```python
from build123d import *

# Parameters (mm, degrees)
SKETCH_1_W          = 97.1
SKETCH_1_H          = 100
EXTRUDE_1_DEPTH     = 1.25
SKETCH_2_W          = 10
SKETCH_2_H          = 10
EXTRUDE_2_DEPTH     = 2.5
CUT_EXTRUDE_2_DEPTH = 3.5
SKETCH_3_R          = 0.75
CUT_EXTRUDE_1_DEPTH = 3.5
FILLET_1_R          = 0.5
SKETCH_6_W          = 77.1
SKETCH_6_H          = 40
CUT_EXTRUDE_3_DEPTH = 3.5
CHAMFER_1_SIZE      = 5
FILLET_2_R          = 1
CUT_EXTRUDE_4_DEPTH = 3.5


with BuildPart() as part:
    # 草图1 → 凸台-拉伸1 (new body, symmetric)
    with BuildSketch(Plane.XY):
        Rectangle(SKETCH_1_W, SKETCH_1_H)
    extrude(amount=EXTRUDE_1_DEPTH, both=True)

    # 草图2 → 凸台-拉伸2 (add)
    with BuildSketch(Plane.XY.offset(1.25)):
        with Locations((-48.55, -40)):
            Rectangle(SKETCH_2_W, SKETCH_2_H)
        with Locations((-48.55, 40)):
            Rectangle(SKETCH_2_W, SKETCH_2_H)
        with Locations((48.55, -40)):
            Rectangle(SKETCH_2_W, SKETCH_2_H)
        with Locations((48.55, 40)):
            Rectangle(SKETCH_2_W, SKETCH_2_H)
    extrude(amount=-EXTRUDE_2_DEPTH)

    # 草图5 → 切除-拉伸2 (cut, through all)
    with BuildSketch(Plane.XY.offset(1.25)):
        Polygon((-38.5, 50), (-38.5, 45), (-36, 45), (-36, 35), (-38.5, 35), (-38.5, 30), (38.5, 30), (38.5, 35), (36, 35), (36, 45), (38.5, 45), (38.5, 50), align=None)
        Polygon((-38.5, -50), (-38.5, -45), (-36, -45), (-36, -35), (-38.5, -35), (-38.5, -30), (38.5, -30), (38.5, -35), (36, -35), (36, -45), (38.5, -45), (38.5, -50), align=None)
    extrude(amount=-CUT_EXTRUDE_2_DEPTH, mode=Mode.SUBTRACT)

    # 草图3 → 切除-拉伸1 (cut, through all)
    with BuildSketch(Plane.XY.offset(1.25)):
        with Locations((-48.55, 34.25)):
            Circle(SKETCH_3_R)
        with Locations((-48.55, 45.75)):
            Circle(SKETCH_3_R)
        with Locations((-48.55, -34.25)):
            Circle(SKETCH_3_R)
        with Locations((-48.55, -45.75)):
            Circle(SKETCH_3_R)
        with Locations((48.55, -34.25)):
            Circle(SKETCH_3_R)
        with Locations((48.55, -45.75)):
            Circle(SKETCH_3_R)
        with Locations((48.55, 34.25)):
            Circle(SKETCH_3_R)
        with Locations((48.55, 45.75)):
            Circle(SKETCH_3_R)
        with Locations((-38.5, 45.75)):
            Circle(SKETCH_3_R)
        with Locations((-38.5, 34.25)):
            Circle(SKETCH_3_R)
        with Locations((-37.75, 30)):
            Circle(SKETCH_3_R)
        with Locations((-37.75, -30)):
            Circle(SKETCH_3_R)
        with Locations((-38.5, -34.25)):
            Circle(SKETCH_3_R)
        with Locations((-38.5, -45.75)):
            Circle(SKETCH_3_R)
        with Locations((38.5, -45.75)):
            Circle(SKETCH_3_R)
        with Locations((38.5, -34.25)):
            Circle(SKETCH_3_R)
        with Locations((37.75, -30)):
            Circle(SKETCH_3_R)
        with Locations((37.75, 30)):
            Circle(SKETCH_3_R)
        with Locations((38.5, 34.25)):
            Circle(SKETCH_3_R)
        with Locations((38.5, 45.75)):
            Circle(SKETCH_3_R)
    extrude(amount=-CUT_EXTRUDE_1_DEPTH, mode=Mode.SUBTRACT)

    # 圆角1
    fillet_1_edges = [part.edges().sort_by_distance(p)[0] for p in [
        (36, 45, 0),
        (36, 35, 0),
        (-36, 35, 0),
        (-36, 45, 0),
        (-36, -45, 0),
        (-36, -35, 0),
        (36, -35, 0),
        (36, -45, 0),
        (-53.55, -35, 0),
        (-53.55, -45, 0),
        (-53.55, 45, 0),
        (-53.55, 35, 0),
        (53.55, -45, 0),
        (53.55, -35, 0),
        (53.55, 35, 0),
        (53.55, 45, 0),
    ]]
    fillet(fillet_1_edges, radius=FILLET_1_R)

    # 草图6 → 切除-拉伸3 (cut, through all)
    with BuildSketch(Plane.XY.offset(1.25)):
        Rectangle(SKETCH_6_W, SKETCH_6_H)
    extrude(amount=-CUT_EXTRUDE_3_DEPTH, mode=Mode.SUBTRACT)

    # 倒角1
    chamfer_1_edges = [part.edges().sort_by_distance(p)[0] for p in [
        (-38.55, -20, 0),
        (-38.55, 20, 0),
        (38.55, 20, 0),
        (38.55, -20, 0),
    ]]
    chamfer(chamfer_1_edges, length=CHAMFER_1_SIZE)

    # 圆角2
    fillet_2_edges = [part.edges().sort_by_distance(p)[0] for p in [
        (33.55, -20, 0),
        (-33.55, -20, 0),
        (-38.55, 15, 0),
        (-38.55, -15, 0),
        (38.55, 15, 0),
        (38.55, -15, 0),
        (-33.55, 20, 0),
        (33.55, 20, 0),
    ]]
    fillet(fillet_2_edges, radius=FILLET_2_R)

    # 草图7 → 切除-拉伸4 (cut, through all)
    with BuildSketch(Plane.XY.offset(1.25)):
        with BuildLine():
            Line((-44.525, -42), (-44.525, 42))
            ThreePointArc((-44.525, 42), (-43.525, 43), (-42.525, 42))
            Line((-42.525, 42), (-42.525, -42))
            ThreePointArc((-42.525, -42), (-43.525, -43), (-44.525, -42))
        make_face()
        with BuildLine():
            Line((44.525, -42), (44.525, 42))
            ThreePointArc((44.525, 42), (43.525, 43), (42.525, 42))
            Line((42.525, 42), (42.525, -42))
            ThreePointArc((42.525, -42), (43.525, -43), (44.525, -42))
        make_face()
    extrude(amount=-CUT_EXTRUDE_4_DEPTH, mode=Mode.SUBTRACT)


solid = part.part
```
Design review of the part built by this model. Coordinates are the model's own, in mm. A direction names the side the tool comes from. Round coordinates to 2 decimals unless told otherwise and drop trailing zeros. Order: outer loops, then holes, each group sorted by start corner. A loop starts at its lowest first (then second) coordinate and runs counter-clockwise, first axis right, second up. Notation, with made-up numbers: (86.25, -18) - (107.25, -18) arc R30 ccw to (107.25, 11) - close; hole circle Ø4 at (-26, -2.75). An arc over 180 degrees is marked (long way). One line per question, with ' | ' between items.
Item 1: Draft analysis for pull direction Y (two halves, no side actions). For faces 1 (the face through (-51, 45, 0)), 2 (the face through (36, 40, 0)), 3 (the face through (36.02, 17.53, 0.02)), state which applies: +Y half, -Y half, draft (parallel to the pull), parting line (faces both ways), or undercut.
Checks:
face 1: +Y half | face 2: draft | face 3: undercut
Item 2: Wall thickness on line 1 (X direction, y = -14.5, z = -0.3) (3 decimals); line 2 (X direction, y = -25, z = 0.15) (3 decimals): over which ranges is each line inside the solid? List them lowest first. Write a range as [from, to].
Checks:
line 1: [-48.55, -44.525], [-42.525, -38.55], [38.55, 42.525], [44.525, 48.55] | line 2: [-48.55, -44.525], [-42.525, 42.525], [44.525, 48.55]
Item 3: Machinability: for faces 4 (the face through (38.5, 32, 0)), 5 (the face through (51, 45, 0)), 6 (the face through (-48.55, 0, 0)), which of the approach directions +Z, -Z, +X, -X, +Y, -Y give a long, thin tool a straight path to every point of the face, cutting with its end or side? Answer none if there is none.
Checks:
face 4: +Z, -Z | face 5: +Z, -Z, +X, +Y | face 6: +Z, -Z, -X
Item 4: Take a section at A-A, the plane y = -22.5. Write out the cut boundary in (x, z) (3 decimals).
Checks:
outline: (-48.55, -1.25) - (-44.525, -1.25) - (-44.525, 1.25) - (-48.55, 1.25) - close; (-42.525, -1.25) - (42.525, -1.25) - (42.525, 1.25) - (-42.525, 1.25) - close; (44.525, -1.25) - (48.55, -1.25) - (48.55, 1.25) - (44.525, 1.25) - close
Item 5: For P1, Ø0.6, axis at x = -37, z = 0.5, coming from the -Y side; P2, Ø0.8, axis at y = -9, z = 0.5, coming from the +X side; P3, Ø1, axis at y = 12.5, z = 1, coming from the -X side, all flat-tipped, find the tip position at first contact; note any pin that passes through.
Checks:
P1: y = -45 | P2: x = 48.55 | P3: x = -48.55
Item 6: Take a section at D-D, the plane z = 0.65. Give the number of separate pieces and of enclosed holes in the cut face, then the cut area to 3 significant figures.
Checks:
separate pieces: 1 | enclosed holes: 3 | area: 3,540 mm²
Item 7: Take a section at C-C, the plane y = 5. Write out the cut boundary in (x, z) (3 decimals), then the cut area to 3 significant figures.
Checks:
outline: (-48.55, -1.25) - (-44.525, -1.25) - (-44.525, 1.25) - (-48.55, 1.25) - close; (-42.525, -1.25) - (-38.55, -1.25) - (-38.55, 1.25) - (-42.525, 1.25) - close; (38.55, -1.25) - (42.525, -1.25) - (42.525, 1.25) - (38.55, 1.25) - close; (44.525, -1.25) - (48.55, -1.25) - (48.55, 1.25) - (44.525, 1.25) - close | area: 40.0 mm²
Item 8: Take a section at B-B, the plane x = 9.5. Write out the cut boundary in (y, z).
Checks:
outline: (-30, -1.25) - (-20, -1.25) - (-20, 1.25) - (-30, 1.25) - close; (20, -1.25) - (30, -1.25) - (30, 1.25) - (20, 1.25) - close
